```python
from build123d import *

# Parameters (mm, degrees)
BOSS_EXTRUDE1_DEPTH = 4.4
BOSS_EXTRUDE2_DEPTH = 16
BOSS_EXTRUDE3_DEPTH = 11
SKETCH2_R           = 2.5
CUT_EXTRUDE1_DEPTH  = 46.664537663
SKETCH3_R           = 3.5
SKETCH3_R_2         = 1.7
SKETCH3_R_3         = 3.648925592
SKETCH3_R_4         = 1.97040034
CUT_EXTRUDE2_DEPTH  = 1
SKETCH3_3_R         = 1.7
SKETCH3_3_R_2       = 1.97040034
CUT_EXTRUDE3_DEPTH  = 46.812771145
FILLET1_R           = 1


with BuildPart() as part:
    # Sketch1 → Boss-Extrude1 (new body)
    with BuildSketch(Plane.XY):
        with BuildLine():
            Line((0, 18), (22.5, 18))
            ThreePointArc((22.5, 18), (40.5, 0), (22.5, -18))
            Line((22.5, -18), (0, -18))
            ThreePointArc((0, -18), (-18, 0), (0, 18))
        make_face()
        with BuildLine():
            ThreePointArc((22.5, -7.6), (30.1, 0), (22.5, 7.6))
            Line((22.5, 7.6), (0, 7.6))
            ThreePointArc((0, 7.6), (-7.6, 0), (0, -7.6))
            Line((0, -7.6), (22.5, -7.6))
        make_face(mode=Mode.SUBTRACT)
    extrude(amount=BOSS_EXTRUDE1_DEPTH)

    # Sketch1_3 → Boss-Extrude2 (add)
    with BuildSketch(Plane.XY):
        with BuildLine():
            Line((0, -7.6), (22.5, -7.6))
            ThreePointArc((22.5, -7.6), (30.1, 0), (22.5, 7.6))
            Line((22.5, 7.6), (0, 7.6))
            ThreePointArc((0, 7.6), (-7.6, 0), (0, -7.6))
        make_face()
        with BuildLine():
            ThreePointArc((22.5, -5), (27.5, 0), (22.5, 5))
            Line((22.5, 5), (0, 5))
            ThreePointArc((0, 5), (-5, 0), (0, -5))
            Line((0, -5), (22.5, -5))
        make_face(mode=Mode.SUBTRACT)
    extrude(amount=BOSS_EXTRUDE2_DEPTH)

    # Sketch1_4 → Boss-Extrude3 (add)
    with BuildSketch(Plane.XY):
        with BuildLine():
            Line((0, -5), (22.5, -5))
            ThreePointArc((22.5, -5), (27.5, 0), (22.5, 5))
            Line((22.5, 5), (0, 5))
            ThreePointArc((0, 5), (-5, 0), (0, -5))
        make_face()
    extrude(amount=BOSS_EXTRUDE3_DEPTH)

    # Sketch2 → Cut-Extrude1 (cut, through all)
    with BuildSketch(Plane.XY.offset(11)):
        Circle(SKETCH2_R)
        with Locations((22.5, 0)):
            Circle(SKETCH2_R)
    extrude(amount=-CUT_EXTRUDE1_DEPTH, mode=Mode.SUBTRACT)

    # Sketch3 → Cut-Extrude2 (cut)
    # profile 1 of 6: a face of its own
    with BuildSketch(Plane.XY.offset(4.4)):
        with Locations((35.5, 0)):
            Circle(SKETCH3_R)
        with Locations((35.5, 0)):
            Circle(SKETCH3_R_2, mode=Mode.SUBTRACT)
    # profile 2 of 6: a face of its own
    with BuildSketch(Plane.XY.offset(4.4)):
        with Locations((-13, 0)):
            Circle(SKETCH3_R_3)
        with Locations((-13, 0)):
            Circle(SKETCH3_R_4, mode=Mode.SUBTRACT)
    # profile 3 of 6: a face of its own
    with BuildSketch(Plane.XY.offset(4.4)):
        with Locations((22.5, -13)):
            Circle(SKETCH3_R)
        with Locations((22.5, -13)):
            Circle(SKETCH3_R_2, mode=Mode.SUBTRACT)
    # profile 4 of 6: a face of its own
    with BuildSketch(Plane.XY.offset(4.4)):
        with Locations((0, 13)):
            Circle(SKETCH3_R_3)
        with Locations((0, 13)):
            Circle(SKETCH3_R_4, mode=Mode.SUBTRACT)
    # profile 5 of 6: a face of its own
    with BuildSketch(Plane.XY.offset(4.4)):
        with Locations((0, -13)):
            Circle(SKETCH3_R_3)
        with Locations((0, -13)):
            Circle(SKETCH3_R_4, mode=Mode.SUBTRACT)
    # profile 6 of 6: a face of its own
    with BuildSketch(Plane.XY.offset(4.4)):
        with Locations((22.5, 13)):
            Circle(SKETCH3_R)
        with Locations((22.5, 13)):
            Circle(SKETCH3_R_2, mode=Mode.SUBTRACT)
    extrude(amount=-CUT_EXTRUDE2_DEPTH, mode=Mode.SUBTRACT)

    # Sketch3_3 → Cut-Extrude3 (cut, through all)
    with BuildSketch(Plane.XY.offset(4.4)):
        with Locations((35.5, 0)):
            Circle(SKETCH3_3_R)
        with Locations((-13, 0)):
            Circle(SKETCH3_3_R_2)
        with Locations((22.5, -13)):
            Circle(SKETCH3_3_R)
        with Locations((0, 13)):
            Circle(SKETCH3_3_R_2)
        with Locations((0, -13)):
            Circle(SKETCH3_3_R_2)
        with Locations((22.5, 13)):
            Circle(SKETCH3_3_R)
    extrude(amount=-CUT_EXTRUDE3_DEPTH, mode=Mode.SUBTRACT)

    # Fillet1
    fillet1_edges = [part.edges().sort_by_distance(p)[0] for p in [
        (11.25, -7.6, 4.4),
        (-7.6, 0, 4.4),
        (11.25, 7.6, 4.4),
        (11.25, 18, 4.4),
        (-18, 0, 4.4),
        (11.25, -18, 4.4),
        (40.5, 0, 4.4),
        (30.1, 0, 4.4),
    ]]
    fillet(fillet1_edges, radius=FILLET1_R)


solid = part.part
```
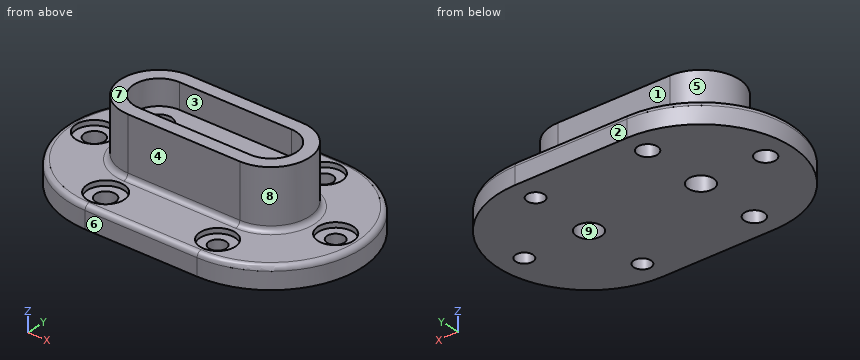
Read the model definition and answer for the solid it produces. Units are mm, in the model's axes. Face numbers are marked on the shaded views. A direction names the side the tool comes from. Coordinates: 2 decimals unless noted, no trailing zeros. Write each loop counter-clockwise with the first axis right and the second up, starting at its lowest first coordinate (ties: lowest second). Pieces come first, ordered by that corner, then holes. Notation, with made-up numbers: (-4, 14) -> (24, 14) arc R15 ccw to (24, 31) -> close; hole circle Ø4 at (-19, 8). An arc over 180 degrees is marked (long way). Answer as a JSON object with one key per item and string values.
Q1. The part is cut by section B-B on x = 13. Give the vertices of the cut face in (y, z).
The answers:
{"outline": "(-18, 0) -> (18, 0) -> (18, 3.4) arc R1 ccw to (17, 4.4) -> (8.6, 4.4) arc R1 cw to (7.6, 5.4) -> (7.6, 16) -> (5, 16) -> (5, 11) -> (-5, 11) -> (-5, 16) -> (-7.6, 16) -> (-7.6, 5.4) arc R1 cw to (-8.6, 4.4) -> (-17, 4.4) arc R1 ccw to (-18, 3.4) -> close"}
Q2. A tool of negligible diameter and unlimited length cuts with its end or side. For the marked faces 1, 2, 3, 4 and 5, from which of +Z, -Z, +X, -X, +Y, -Y can it reach the whole face along a straight path? Write none if from no direction.
The answers:
{"face 1": "+Z, +X, -X, +Y", "face 2": "+Z, -Z, +X, -X, +Y", "face 3": "+Z", "face 4": "+Z, +X, -X, -Y", "face 5": "+Z, -X"}
Q3. The part is cut by section C-C on y = 13. Give the number of separate pieces and of enclosed holes in the cut face, then the cut area to 3 significant figures.
The answers:
{"separate pieces": "3", "enclosed holes": "0", "area": "169 mm2"}
Q4. Consider line 1 (Y direction, x = 8.5, z = 14.5); line 2 (Z direction, x = 26, y = -8); line 3 (Z direction, x = 4, y = 2). Determine where each line is inside the solid, lowest interval first. Write a range as [from, to].
The answers:
{"line 1": "y = [-7.6, -5], [5, 7.6]", "line 2": "z = [0, 4.4]", "line 3": "z = [0, 11]"}
Q5. The part is cut by section A-A on z = 11.75. Give the vertices of the cut face in (x, y).
The answers:
{"outline": "(0, -7.6) -> (22.5, -7.6) arc R7.6 ccw to (22.5, 7.6) -> (0, 7.6) arc R7.6 ccw to start; hole (0, -5) -> (22.5, -5) arc R5 ccw to (22.5, 5) -> (0, 5) arc R5 ccw to start"}
Q6. Determine the mould class of the marked faces 6, 7, 8 and 9 for opening direction Y: pulls with the +Y half, pulls with the -Y half, needs draft (parallel to the pull), parting line crosses it, or undercut.
The answers:
{"face 6": "pulls with the -Y half", "face 7": "needs draft", "face 8": "parting line crosses it", "face 9": "undercut"}
Q7. Flat-ended cylindrical pins translate along their axes: pin 1 Ø1.5 at (y, z) = (1, 13) entering from +X; pin 2 Ø4 at (x, y) = (22.5, 0) entering from +Z; pin 3 Ø4 at (y, z) = (-7.5, 6) entering from -X; pin 4 Ø5.5 at (x, y) = (21, 14.5) entering from +Z. Find the tip coordinate at first contact, or state that the pin passes through.
The answers:
{"pin 1": "stops at x = 30.1", "pin 2": "passes through", "pin 3": "stops at x = -16.33", "pin 4": "stops at z = 4.4"}
